Geometry: final body of the model. Coordinates: model frame, mm. A direction names the side the tool comes from. Give positions to 0.01 mm unless a question says otherwise; leave off trailing zeros. Write each loop counter-clockwise with the first axis right and the second up, starting at its lowest first coordinate (ties: lowest second). Pieces come first, ordered by that corner, then holes.
from build123d import *

# Parameters (mm, degrees)
SKETCH2_W         = 18.3
SKETCH2_H         = 2.8
SLOT_DEPTH        = 4.4
SKETCH3_W         = 2.17
SKETCH3_H         = 11.24
SKETCH4_W         = 1.085
SKETCH4_H         = 1.085
CIRPATTERN1_COUNT = 2
CIRPATTERN1_ANGLE = 90


with BuildPart() as part:
    # BodySke → Base-Revolve (revolve)
    with BuildSketch(Plane.XY):
        with BuildLine():
            Line((0, 0), (42.298786444, 0))
            Line((42.298786444, 0), (42.298786444, 5))
            Line((42.298786444, 5), (7.298786444, 5))
            Line((7.298786444, 5), (3.148786444, 9.15))
            Line((3.148786444, 9.15), (1.907441795, 9.15))
            ThreePointArc((1.907441795, 9.15), (0.481931585, 4.673350891), (0, 0))
        make_face()
    revolve(axis=Axis((-15.875, 0, 0), (1, 0, 0)))

    # Sketch2 → Slot (cut)
    with BuildSketch(Plane(origin=(0, 0, 0), x_dir=(0, 0, -1), z_dir=(1, 0, 0))):
        Rectangle(SKETCH2_W, SKETCH2_H)
    extrude(amount=SLOT_DEPTH, mode=Mode.SUBTRACT)

    # Sketch3 → Cross section 0
    with BuildSketch(Plane(origin=(0, 0, 0), x_dir=(0, 0, -1), z_dir=(1, 0, 0))):
        Rectangle(SKETCH3_W, SKETCH3_H)
    # Sketch4 → Cross section 1
    with BuildSketch(Plane(origin=(7.15, 0, 0), x_dir=(0, 0, -1), z_dir=(1, 0, 0))):
        Rectangle(SKETCH4_W, SKETCH4_H)
    cross = loft(mode=Mode.SUBTRACT)

    # CirPattern1: Cross ×2 about axis
    cirpattern1_axis = Axis((0, 0, 0), (1, 0, 0))
    for i in range(1, CIRPATTERN1_COUNT):
        add(cross.rotate(cirpattern1_axis, i * CIRPATTERN1_ANGLE / (CIRPATTERN1_COUNT - 1)), mode=Mode.SUBTRACT)


solid = part.part
Q1. Pull-direction query (Y, two-part tool) for faces 1 (the cylindrical face through (2.52, -9.15, 0.18)), 2 (the conical face through (7.039, -1.14, -5.135)), 3 (the flat face through (4.4, 0, -4)), 4 (the flat face through (42.299, 0, 0)); classes: released by +Y, released by -Y, zero draft, split by the parting line, or undercut.
Filled sheet:
face 1: released by -Y
face 2: split by the parting line
face 3: undercut
face 4: zero draft
Q2. Access query for faces 5 (the cylindrical face through (24.55, -1.08, -4.88)), 6 (the flat face through (7.15, 0, 0)), 7 (the flat face through (3, -1.4, -5)). Directions: +Z, -Z, +X, -X, +Y, -Y. A direction counts if a zero-diameter tool reaches every point of the face in a straight line with its end or side. Return the directions, or none.
Filled sheet:
face 5: +X
face 6: -X
face 7: +Z, -Z, -X
Q3. Pin query (flat end, axial travel): P1, Ø3, axis at x = 19, y = 1.5, coming from the -Z side; P2, Ø5, axis at x = 3, z = -4, coming from the +Y side; P3, Ø1.2, axis at y = 0, z = 0, coming from the -X side. Return the tip coordinate at first contact, or that it passes through.
Filled sheet:
P1: stops at z = -5
P2: stops at y = 9.03
P3: stops at x = 7.07
Q4. Section A-A on x = 23.5. Output: boundary loops of the cut face in (y, z), plus the area to 3 significant figures.
Filled sheet:
outline: circle Ø10 at (0, 0)
area: 78.5 mm2
Q5. Ray query, line 1 along Y through (x, z) = (4, -5); line 2 along Z through (x, y) = (38, 0.25); line 3 along X through (y, z) = (-1.25, -1). Return the intervals inside material, ascending.
Filled sheet:
line 1: y = -6.62 to -1.4, 1.4 to 6.62
line 2: z = -4.99 to 4.99
line 3: x = 4.4 to 42.3
